from build123d import *

# Parameters (mm, degrees)
SKETCH1_R           = 3
SKETCH1_R_2         = 0.815869739
BOSS_EXTRUDE1_DEPTH = 18
SKETCH2_R           = 6
CUT_EXTRUDE1_DEPTH  = 6


with BuildPart() as part:
    # Sketch1 → Boss-Extrude1 (new body)
    with BuildSketch(Plane(origin=(0, 0, 0), x_dir=(1, 0, 0), z_dir=(0, 1, 0))):
        with BuildLine():
            Line((-45, 13), (-45, -13))
            ThreePointArc((-45, -13), (-44.414213562, -14.414213562), (-43, -15))
            Line((-43, -15), (43, -15))
            ThreePointArc((43, -15), (44.414213562, -14.414213562), (45, -13))
            Line((45, -13), (45, 13))
            ThreePointArc((45, 13), (44.414213562, 14.414213562), (43, 15))
            Line((43, 15), (-43, 15))
            ThreePointArc((-43, 15), (-44.414213562, 14.414213562), (-45, 13))
        make_face()
        with Locations((-32.5, 0)):
            Circle(SKETCH1_R, mode=Mode.SUBTRACT)
        with Locations((32.5, 0)):
            Circle(SKETCH1_R, mode=Mode.SUBTRACT)
        with Locations((-31.184130261, 4.910892723)):
            Circle(SKETCH1_R_2, mode=Mode.SUBTRACT)
        with Locations((-33.815869739, 4.910892723)):
            Circle(SKETCH1_R_2, mode=Mode.SUBTRACT)
        with Locations((-36.095022984, 3.595022984)):
            Circle(SKETCH1_R_2, mode=Mode.SUBTRACT)
        with Locations((-37.410892723, 1.315869739)):
            Circle(SKETCH1_R_2, mode=Mode.SUBTRACT)
        with Locations((-37.410892723, -1.315869739)):
            Circle(SKETCH1_R_2, mode=Mode.SUBTRACT)
        with Locations((-36.095022984, -3.595022984)):
            Circle(SKETCH1_R_2, mode=Mode.SUBTRACT)
        with Locations((-33.815869739, -4.910892723)):
            Circle(SKETCH1_R_2, mode=Mode.SUBTRACT)
        with Locations((-31.184130261, -4.910892723)):
            Circle(SKETCH1_R_2, mode=Mode.SUBTRACT)
        with Locations((-28.904977016, -3.595022984)):
            Circle(SKETCH1_R_2, mode=Mode.SUBTRACT)
        with Locations((-27.589107277, -1.315869739)):
            Circle(SKETCH1_R_2, mode=Mode.SUBTRACT)
        with Locations((-27.589107277, 1.315869739)):
            Circle(SKETCH1_R_2, mode=Mode.SUBTRACT)
        with Locations((-28.904977016, 3.595022984)):
            Circle(SKETCH1_R_2, mode=Mode.SUBTRACT)
        with Locations((31.184130261, 4.910892723)):
            Circle(SKETCH1_R_2, mode=Mode.SUBTRACT)
        with Locations((33.815869739, 4.910892723)):
            Circle(SKETCH1_R_2, mode=Mode.SUBTRACT)
        with Locations((36.095022984, 3.595022984)):
            Circle(SKETCH1_R_2, mode=Mode.SUBTRACT)
        with Locations((37.410892723, 1.315869739)):
            Circle(SKETCH1_R_2, mode=Mode.SUBTRACT)
        with Locations((37.410892723, -1.315869739)):
            Circle(SKETCH1_R_2, mode=Mode.SUBTRACT)
        with Locations((36.095022984, -3.595022984)):
            Circle(SKETCH1_R_2, mode=Mode.SUBTRACT)
        with Locations((33.815869739, -4.910892723)):
            Circle(SKETCH1_R_2, mode=Mode.SUBTRACT)
        with Locations((31.184130261, -4.910892723)):
            Circle(SKETCH1_R_2, mode=Mode.SUBTRACT)
        with Locations((28.904977016, -3.595022984)):
            Circle(SKETCH1_R_2, mode=Mode.SUBTRACT)
        with Locations((27.589107277, -1.315869739)):
            Circle(SKETCH1_R_2, mode=Mode.SUBTRACT)
        with Locations((27.589107277, 1.315869739)):
            Circle(SKETCH1_R_2, mode=Mode.SUBTRACT)
        with Locations((28.904977016, 3.595022984)):
            Circle(SKETCH1_R_2, mode=Mode.SUBTRACT)
    extrude(amount=BOSS_EXTRUDE1_DEPTH)

    # Sketch2 → Cut-Extrude1 (cut)
    with BuildSketch(Plane(origin=(0, 18, 0), x_dir=(1, 0, 0), z_dir=(0, 1, 0))):
        with Locations((32.5, 0)):
            Circle(SKETCH2_R)
        with Locations((-32.5, 0)):
            Circle(SKETCH2_R)
    extrude(amount=-CUT_EXTRUDE1_DEPTH, mode=Mode.SUBTRACT)


solid = part.part
CAD build for the part. Positions are in the model's coordinates, mm. A direction names the side the tool comes from. Round coordinates to 2 decimals unless told otherwise and drop trailing zeros. Write each loop counter-clockwise with the first axis right and the second up, starting at its lowest first coordinate (ties: lowest second). Pieces come first, ordered by that corner, then holes.
(1) Slice it at B-B, the plane y = 7. Count the separate pieces of the cut face and the enclosed holes in it, and give its area (3 significant figures).
(2) Probe line 1 along X through (y, z) = (14.25, -2); line 2 along X through (y, z) = (4.5, 0); line 3 along Z through (x, y) = (32.5, 4.75). List the from-to ranges inside material, lowest first.
(3) Mould opens along Z. For faces 1 (the face through (-1, 9, 15)), 2 (the face through (1, 9, -15)), 3 (the face through (-33.038, 5.916, 4.666)) say: pulls with the +Z half, pulls with the -Z half, needs draft (parallel to the pull), parting line crosses it, or undercut.
(4) 3-axis set-ups, long thin cutter, end or side, ignore diameter. For faces 4 (the face through (36.596, 5.916, 1.28)), 5 (the face through (34, 12, -3)): which of +Z, -Z, +X, -X, +Y, -Y reach the whole face in a straight line?
(5) Slice it at A-A, the plane y = 14. Write the cut outline in (x, z), and give its area (3 significant figures).
From the geometry:
1. separate pieces: 1
1. enclosed holes: 26
1. area: 2,590 mm2
2. line 1: x = -45 to -38.16, -26.84 to 26.84, 38.16 to 45
2. line 2: x = -45 to -35.5, -29.5 to 29.5, 35.5 to 45
2. line 3: z = -15 to -3, 3 to 15
3. face 1: pulls with the +Z half
3. face 2: pulls with the -Z half
3. face 3: undercut
4. face 4: +Y, -Y
4. face 5: +Y
5. outline: (-45, -13) arc R2 ccw to (-43, -15) - (43, -15) arc R2 ccw to (45, -13) - (45, 13) arc R2 ccw to (43, 15) - (-43, 15) arc R2 ccw to (-45, 13) - close; hole circle Ø12 at (-32.5, 0); hole circle Ø12 at (32.5, 0)
5. area: 2,470 mm2
